Check sheet for the modelled part. Datum: model origin and axes. Units: mm. Face numbers are marked on the shaded views. A direction names the side the tool comes from. Give positions to 0.01 mm unless a question says otherwise; leave off trailing zeros. Loops run counter-clockwise (first coordinate to the right, second up) from the corner with the lowest first, then second, coordinate; pieces in that order, holes last. Notation, with made-up numbers: (62, 48) - (100, 48) arc R11 ccw to (100, 56) - close; hole circle Ø7 at (86.5, 71). An arc over 180 degrees is marked (long way). Use CSV: the item, a comma, the result in double quotes.
from build123d import *

# Parameters (mm, degrees)
F0_W   = 24.017472
F0_H   = 17.362025
F0_W_2 = 11.285316
F0_H_2 = 15.625823
F2_R   = 5.08
F3_R   = 0.508


with BuildPart() as f1:
    # F0 (on Front) → F1 (revolve)
    with BuildSketch(Plane.XZ):
        with Locations((23.294052, 24.451518)):
            Rectangle(F0_W, F0_H)
        with Locations((5.642658, 40.945442)):
            Rectangle(F0_W_2, F0_H_2)
        with Locations((5.642658, 24.451518)):
            Rectangle(F0_W_2, F0_H)
    revolve(axis=Axis((42.247593, 0, 0), (1, 0, 0)))

    # F2
    f2_edges = [f1.edges().sort_by_distance(p)[0] for p in [
        (11.285316, 0, -33.132531),
    ]]
    fillet(f2_edges, radius=F2_R)

    # F3
    f3_edges = [f1.edges().sort_by_distance(p)[0] for p in [
        (35.302788, 0, -33.132531),
    ]]
    fillet(f3_edges, radius=F3_R)


solid = f1.part
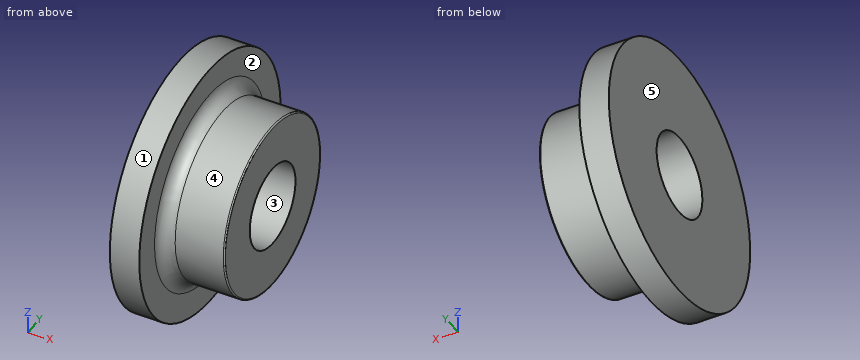
1. Set-up check for the marked faces 1 and 2: record each of +Z, -Z, +X, -X, +Y, -Y from which the full face is reachable in a straight line by a thin tool's end or side.
Completed:
face 1,"+X, -X"
face 2,"+X"
2. Scan lines: line 1 along Z through (x, y) = (26, 0); line 2 along Z through (x, y) = (8, 0). Record each from-to range of solid material in increasing order.
Completed:
line 1,"z = -33.13 to -15.77, 15.77 to 33.13"
line 2,"z = -48.76 to -15.77, 15.77 to 48.76"
3. Go/stop test with flat-tipped pins: pin 1 Ø12 at (x, y) = (27, -1) entering from +Z; pin 2 Ø2 at (x, y) = (8.5, 22.5) entering from +Z; pin 3 Ø8 at (x, y) = (27.5, -21) entering from +Z. Record where each tip stops, or that it passes through.
Completed:
pin 1,"stops at z = 33.13"
pin 2,"stops at z = 43.76"
pin 3,"stops at z = 28.44"
4. Sectioned sample at A-A, the plane z = 0. Record the boundary of the cut face in (x, y), and give its area (3 significant figures).
Completed:
outline,"(0, -48.76) - (11.29, -48.76) - (11.29, -38.21) arc R5.08 cw to (16.37, -33.13) - (34.79, -33.13) arc R0.51 ccw to (35.3, -32.62) - (35.3, -15.77) - (0, -15.77) - close; (0, 15.77) - (35.3, 15.77) - (35.3, 32.62) arc R0.51 ccw to (34.79, 33.13) - (16.37, 33.13) arc R5.08 cw to (11.29, 38.21) - (11.29, 48.76) - (0, 48.76) - close"
area,"1,590 mm²"
5. Sectioned sample at C-C, the plane x = 21.5. Record the boundary of the cut face in (y, z).
Completed:
outline,"circle Ø66.27 at (0, 0); hole circle Ø31.54 at (0, 0)"
6. Release check for a two-part mould opening along Z. For the marked faces 3, 4 and 5 record: released by +Z, released by -Z, zero draft, split by the parting line, or undercut.
Completed:
face 3,"undercut"
face 4,"split by the parting line"
face 5,"zero draft"
7. Sectioned sample at D-D, the plane x = 5. Record the boundary of the cut face in (y, z), and give its area (3 significant figures).
Completed:
outline,"circle Ø97.52 at (0, 0); hole circle Ø31.54 at (0, 0)"
area,"6,690 mm²"
